from build123d import *

# Parameters (mm, degrees)
SKETCH1_W           = 9
SKETCH1_H           = 3.175
SKETCH1_W_2         = 12
SKETCH1_H_2         = 12
SKETCH1_W_3         = 6
SKETCH1_H_3         = 3.125
SKETCH1_W_4         = 3.175
SKETCH1_H_4         = 6
BOSS_EXTRUDE1_DEPTH = 1.5875


with BuildPart() as part:
    # Sketch1 → Boss-Extrude1 (new, symmetric)
    with BuildSketch(Plane.XY):
        Polygon((54.175, 4.5), (51, 4.5), (51, 13.5), (54.175, 13.5), (54.175, 22.5), (51, 22.5), (51, 31.5), (-51, 31.5), (-51, 22.5), (-54.175, 22.5), (-54.175, 13.5), (-51, 13.5), (-51, 4.5), (-54.175, 4.5), (-54.175, -4.5), (-51, -4.5), (-51, -13.5), (-54.175, -13.5), (-54.175, -22.5), (-51, -22.5), (-51, -31.5), (51, -31.5), (51, -22.5), (54.175, -22.5), (54.175, -13.5), (51, -13.5), (51, -4.5), (54.175, -4.5), align=None)
        with Locations((34, 28)):
            Rectangle(SKETCH1_W, SKETCH1_H, mode=Mode.SUBTRACT)
        with Locations((34, 16.5)):
            Rectangle(SKETCH1_W_2, SKETCH1_H_2, mode=Mode.SUBTRACT)
        with Locations((34, 5)):
            Rectangle(SKETCH1_W, SKETCH1_H, mode=Mode.SUBTRACT)
        with Locations((34, 0)):
            Rectangle(SKETCH1_W_3, SKETCH1_H_3, mode=Mode.SUBTRACT)
        with Locations((34, -16.5)):
            Rectangle(SKETCH1_W_2, SKETCH1_H_2, mode=Mode.SUBTRACT)
        with Locations((44.5875, 8)):
            Rectangle(SKETCH1_W_4, SKETCH1_H_4, mode=Mode.SUBTRACT)
        with Locations((44.5875, 16.5)):
            Rectangle(SKETCH1_W_4, SKETCH1_H_4, mode=Mode.SUBTRACT)
        with Locations((44.5875, 25)):
            Rectangle(SKETCH1_W_4, SKETCH1_H_4, mode=Mode.SUBTRACT)
        with Locations((23.4125, 25)):
            Rectangle(SKETCH1_W_4, SKETCH1_H_4, mode=Mode.SUBTRACT)
        with Locations((17, 21)):
            Rectangle(SKETCH1_W_4, SKETCH1_H_4, mode=Mode.SUBTRACT)
        with Locations((-17, -21)):
            Rectangle(SKETCH1_W_4, SKETCH1_H_4, mode=Mode.SUBTRACT)
        with Locations((17, -21)):
            Rectangle(SKETCH1_W_4, SKETCH1_H_4, mode=Mode.SUBTRACT)
        with Locations((-34, 0)):
            Rectangle(SKETCH1_W_3, SKETCH1_H_3, mode=Mode.SUBTRACT)
        with Locations((-17, 0)):
            Rectangle(SKETCH1_W_4, SKETCH1_H_4, mode=Mode.SUBTRACT)
        with Locations((-17, 21)):
            Rectangle(SKETCH1_W_4, SKETCH1_H_4, mode=Mode.SUBTRACT)
        with Locations((17, 0)):
            Rectangle(SKETCH1_W_4, SKETCH1_H_4, mode=Mode.SUBTRACT)
        with Locations((23.4125, 8)):
            Rectangle(SKETCH1_W_4, SKETCH1_H_4, mode=Mode.SUBTRACT)
        with Locations((23.4125, 16.5)):
            Rectangle(SKETCH1_W_4, SKETCH1_H_4, mode=Mode.SUBTRACT)
    extrude(amount=BOSS_EXTRUDE1_DEPTH, both=True)


solid = part.part
The listing builds one solid part. Answer for the finished solid, in the listing's coordinates (mm). A direction names the side the tool comes from. Give positions to 0.01 mm unless a question says otherwise; leave off trailing zeros. Order: outer loops, then holes, each group sorted by start corner. A loop starts at its lowest first (then second) coordinate and runs counter-clockwise, first axis right, second up. Notation, with made-up numbers: (46, 19.5) - (53, 19.5) arc R19 ccw to (53, 47.5) - close; hole circle Ø11 at (21, 44). An arc over 180 degrees is marked (long way). One line per item, written item: value. Start each with the question number.
1) Find the intervals of material crossed by L1, parallel to Y at x = 34, z = -1.2; L2, parallel to X at y = 8, z = 0.2 (3 decimals); L3, parallel to X at y = 23.5, z = 0.3 (1 decimal), in increasing order.
2) Given pin 1 Ø1.6 at (x, z) = (-53.5, 0.5) entering from -Y, flat-ended and moving along its own axis, determine where the tip first touches the part or whether it passes through.
3) The mould has two halves that part along Y. Classify faces 4 (the face through (51, 27, 0)), 5 (the face through (38.5, 5, 0)): released by +Y, released by -Y, zero draft, split by the parting line, or undercut.
4) A cutting plane is placed at A-A on y = -19.5. Give the vertices of the cut face in (x, z) (1 decimal).
5) A cutting plane is placed at B-B on z = -0.15. State how many separate pieces and enclosed holes the cut face has, then the cut area to 3 significant figures.
6) A tool of negligible diameter and unlimited length cuts with its end or side. For faces 1 (the face through (23, 13.5, 0)), 2 (the face through (53, -13.5, 0)), 3 (the face through (-54.175, 0, 0)), from which of +Z, -Z, +X, -X, +Y, -Y can it reach the whole face along a straight path? Write none if from no direction.
Answer sheet:
1. L1: y = -31.5 to -22.5, -10.5 to -1.56, 1.56 to 3.41, 6.59 to 10.5, 22.5 to 26.41, 29.59 to 31.5
1. L2: x = -51 to 21.825, 25 to 43, 46.175 to 51
1. L3: x = -51 to -18.6, -15.4 to 15.4, 18.6 to 21.8, 25 to 43, 46.2 to 51
2. pin 1: stops at y = -22.5
3. face 4: zero draft
3. face 5: undercut
4. outline: (-54.2, -1.6) - (-18.6, -1.6) - (-18.6, 1.6) - (-54.2, 1.6) - close; (-15.4, -1.6) - (15.4, -1.6) - (15.4, 1.6) - (-15.4, 1.6) - close; (18.6, -1.6) - (28, -1.6) - (28, 1.6) - (18.6, 1.6) - close; (40, -1.6) - (54.2, -1.6) - (54.2, 1.6) - (40, 1.6) - close
5. separate pieces: 1
5. enclosed holes: 18
5. area: 5,990 mm2
6. face 1: +Z, -Z
6. face 2: +Z, -Z, +X
6. face 3: +Z, -Z, -X, +Y, -Y
